CAD build for the part. Positions are in the model's coordinates, mm. A direction names the side the tool comes from. Coordinates: 2 decimals unless noted, no trailing zeros. Loops run counter-clockwise (first coordinate to the right, second up) from the corner with the lowest first, then second, coordinate; pieces in that order, holes last. Notation, with made-up numbers: (75.5, 46.5) -> (107.5, 46.5) arc R23 cw to (107.5, 68.5) -> close; hole circle Ø9 at (61, -27). An arc over 180 degrees is marked (long way). Answer as a JSON object with one key per item and string values. Group by question number.
from build123d import *

# Parameters (mm, degrees)
CYLINDER003001001005001001_R     = 3.5
CYLINDER003001001005001001_DEPTH = 2
CYLINDER003001001004002_R        = 1
CYLINDER003001001004002_DEPTH    = 5
CYLINDER003001001004001001_R     = 1
CYLINDER003001001004001001_DEPTH = 5
CYLINDER003001001005001_R        = 6.5
CYLINDER003001001005001_DEPTH    = 2
BOX002_W                         = 10
BOX002_H                         = 6
BOX002_DEPTH                     = 2
CYLINDER003001001004_R           = 2
CYLINDER003001001004_DEPTH       = 3
CYLINDER003001001004001_R        = 2
CYLINDER003001001004001_DEPTH    = 3
CYLINDER003001001005_R           = 20
CYLINDER003001001005_DEPTH       = 2


with BuildPart() as cylinder013:
    # Cylinder003001001005001001 → Cylinder003001001005001001 (new body)
    with BuildSketch(Plane(origin=(12, 6, 21), x_dir=(1, 0, 0), z_dir=(0, 0, 1))):
        Circle(CYLINDER003001001005001001_R)
    extrude(amount=CYLINDER003001001005001001_DEPTH)


with BuildPart() as cylinder014:
    # Cylinder003001001004002 → Cylinder003001001004002 (new body)
    with BuildSketch(Plane(origin=(-2.5, 6, 16.4), x_dir=(1, 0, 0), z_dir=(0, 0, 1))):
        Circle(CYLINDER003001001004002_R)
    extrude(amount=CYLINDER003001001004002_DEPTH)


with BuildPart() as cylinder015:
    # Cylinder003001001004001001 → Cylinder003001001004001001 (new body)
    with BuildSketch(Plane(origin=(25.5, 6, 16.4), x_dir=(1, 0, 0), z_dir=(0, 0, 1))):
        Circle(CYLINDER003001001004001001_R)
    extrude(amount=CYLINDER003001001004001001_DEPTH)


with BuildPart() as fusion009:
    # Cylinder003001001005001 → Cylinder003001001005001 (new body)
    with BuildSketch(Plane(origin=(6, 6, 21), x_dir=(1, 0, 0), z_dir=(0, 0, 1))):
        Circle(CYLINDER003001001005001_R)
    extrude(amount=CYLINDER003001001005001_DEPTH)

    # Fusion009: union Cylinder013, Cylinder014, Cylinder015
    add(cylinder013.part)
    add(cylinder014.part)
    add(cylinder015.part)


with BuildPart() as box002:
    # Box002 → Box002 (new body)
    with BuildSketch(Plane(origin=(18, 3, 21), x_dir=(1, 0, 0), z_dir=(0, 0, 1))):
        with Locations((5, 3)):
            Rectangle(BOX002_W, BOX002_H)
    extrude(amount=BOX002_DEPTH)


with BuildPart() as cylinder009:
    # Cylinder003001001004 → Cylinder003001001004 (new body)
    with BuildSketch(Plane(origin=(-2.5, 6, 18.4), x_dir=(1, 0, 0), z_dir=(0, 0, 1))):
        Circle(CYLINDER003001001004_R)
    extrude(amount=CYLINDER003001001004_DEPTH)


with BuildPart() as cylinder010:
    # Cylinder003001001004001 → Cylinder003001001004001 (new body)
    with BuildSketch(Plane(origin=(25.5, 6, 18.4), x_dir=(1, 0, 0), z_dir=(0, 0, 1))):
        Circle(CYLINDER003001001004001_R)
    extrude(amount=CYLINDER003001001004001_DEPTH)


with BuildPart() as guide1:
    # Cylinder003001001005 → Cylinder003001001005 (new body)
    with BuildSketch(Plane(origin=(6, 6, 21), x_dir=(1, 0, 0), z_dir=(0, 0, 1))):
        Circle(CYLINDER003001001005_R)
    extrude(amount=CYLINDER003001001005_DEPTH)

    # Fusion008: union Box002, Cylinder009, Cylinder010
    add(box002.part)
    add(cylinder009.part)
    add(cylinder010.part)

    # Cut002: cut Fusion009
    add(fusion009.part, mode=Mode.SUBTRACT)


solid = guide1.part
Item 1: Band-saw the part on A-A, the plane x = 6. List the corners of the cut face in (y, z), and give its area (3 significant figures).
Item 2: Flat gauge pins, fed straight in: P1, Ø2, axis at x = 4, y = -3, coming from the -Z side; P2, Ø1, axis at y = 7.5, z = 21, coming from the -X side (3 decimals); P3, Ø1, axis at x = 27, z = 22.5, coming from the -Y side. Where does each tip first touch, or does it go through?
Item 3: Band-saw the part on B-B, the plane z = 20. List the corners of the cut face in (x, y).
Item 4: Drill centre lines: L1, parallel to Y at x = 6, z = 22.4; L2, parallel to X at y = 6, z = 20.2; L3, parallel to Y at x = -2.5, z = 19.45. Where is each one in solid material? Low to high.
Item 5: Band-saw the part on D-D, the plane x = 15. List the corners of the cut face in (y, z), and give its area (3 significant figures).
Item 6: Band-saw the part on C-C, the plane x = -2.5. List the corners of the cut face in (y, z).
Item 7: Pull direction X, two halves, no side cores. Call faces 4 (the flat face through (28, 6, 22)), 5 (the flat face through (27, 9, 22)), 6 (the cylindrical face through (23.502, 6.088, 19.682)), 7 (the cylindrical face through (25.37, 6.99, 19.88)): +X half, -X half, draft (parallel to the pull), parting line (faces both ways), or undercut.
Item 8: 3-axis set-ups, long thin cutter, end or side, ignore diameter. For faces 1 (the flat face through (27, 3, 22)), 2 (the cylindrical face through (-2.76, 7.983, 19.682)), 3 (the flat face through (26.4, 5.1, 18.4)): which of +Z, -Z, +X, -X, +Y, -Y reach the whole face in a straight line?
Reply:
{
 "1": {"outline": "(-14, 21) -> (-0.5, 21) -> (-0.5, 23) -> (-14, 23) -> close; (12.5, 21) -> (26, 21) -> (26, 23) -> (12.5, 23) -> close", "area": "54.0 mm²"},
 "2": {"P1": "z = 21", "P2": "x = -13.975", "P3": "y = 3"},
 "3": {"outline": "circle Ø4 at (-2.5, 6); circle Ø4 at (25.5, 6); hole circle Ø2 at (-2.5, 6); hole circle Ø2 at (25.5, 6)"},
 "4": {"L1": "-14 to -0.5, 12.5 to 26", "L2": "-4.5 to -3.5, -1.5 to -0.5, 23.5 to 24.5, 26.5 to 27.5", "L3": "4 to 5, 7 to 8"},
 "5": {"outline": "(-11.86, 21) -> (4.2, 21) -> (4.2, 23) -> (-11.86, 23) -> close; (7.8, 21) -> (23.86, 21) -> (23.86, 23) -> (7.8, 23) -> close", "area": "64.2 mm²"},
 "6": {"outline": "(-12.1, 21) -> (4, 21) -> (4, 18.4) -> (5, 18.4) -> (5, 21.4) -> (7, 21.4) -> (7, 18.4) -> (8, 18.4) -> (8, 21) -> (24.1, 21) -> (24.1, 23) -> (-12.1, 23) -> close"},
 "7": {"face 4": "+X half", "face 5": "draft", "face 6": "undercut", "face 7": "undercut"},
 "8": {"face 1": "+Z, -Z, +X, -Y", "face 2": "-Z", "face 3": "-Z, +X, -X, +Y, -Y"}
}
